CAD build for the part. Positions are in the model's coordinates, mm. A direction names the side the tool comes from. Give positions to 0.01 mm unless a question says otherwise; leave off trailing zeros. Loops run counter-clockwise (first coordinate to the right, second up) from the corner with the lowest first, then second, coordinate; pieces in that order, holes last. Notation, with made-up numbers: M -35.75,58 L -2.75,58 A28 ccw -2.75,92 Z; hole C -20.5,0 d11. An arc over 180 degrees is marked long. One line per question, with ' | ' between items.
```python
from build123d import *

# Parameters (mm, degrees)
EXTRUDE_1_DEPTH     = 300
CUT_EXTRUDE_1_DEPTH = 305.46017802


with BuildPart() as part:
    # 草图1 → 凸台-拉伸1 (new body)
    with BuildSketch(Plane(origin=(0, 0, 0), x_dir=(1, 0, 0), z_dir=(0, 1, 0))):
        Polygon((0, 0), (0, 50), (14, 50), (14, 48), (2, 48), (2, 2), (14, 2), (14, 0), align=None)
    extrude(amount=EXTRUDE_1_DEPTH)

    # 草图2 → 切除-拉伸1 (cut, through all)
    with BuildSketch(Plane.ZY):
        with BuildLine():
            Line((-7, 274), (-7, 26))
            ThreePointArc((-7, 26), (-25, 8), (-43, 26))
            Line((-43, 26), (-43, 274))
            ThreePointArc((-43, 274), (-25, 292), (-7, 274))
        make_face()
    extrude(amount=-CUT_EXTRUDE_1_DEPTH, mode=Mode.SUBTRACT)


solid = part.part
```
Item 1: 3-axis set-ups, long thin cutter, end or side, ignore diameter. For faces 1 (the flat face through (8, 148, -2)), 2 (the cylindrical face through (1, 8, -25)), 3 (the flat face through (7, 148, 0)): which of +Z, -Z, +X, -X, +Y, -Y reach the whole face in a straight line?
Conclusion:
face 1: +X, +Y, -Y | face 2: +X, -X | face 3: +Z, +X, -X, +Y, -Y
Item 2: Mould opens along Y. For faces 4 (the flat face through (8, 148, -48)), 5 (the flat face through (1.8, 300, -23.3)), 6 (the cylindrical face through (1, 292, -25)), 7 (the flat face through (1.8, 0, -23.3)) say: pulls with the +Y half, pulls with the -Y half, needs draft (parallel to the pull), parting line crosses it, or undercut.
Conclusion:
face 4: needs draft | face 5: pulls with the +Y half | face 6: undercut | face 7: pulls with the -Y half
Item 3: Saw through at B-B on y = 253. Give the cut face in (x, z).
Conclusion:
outline: M 0,-50 L 14,-50 L 14,-48 L 2,-48 L 2,-43 L 0,-43 Z; M 0,-7 L 2,-7 L 2,-2 L 14,-2 L 14,0 L 0,0 Z
Item 4: Drill centre lines: line 1 along Z through (x, y) = (8.75, 268); line 2 along Z through (x, y) = (1, 80); line 3 along Y through (x, z) = (1.5, -22). Where is each one in solid material? Low to high. Write a range as [from, to].
Conclusion:
line 1: [-50, -48], [-2, 0] | line 2: [-50, -43], [-7, 0] | line 3: [0, 8.25], [291.75, 300]
Item 5: Saw through at C-C on z = -25. Give the cut face in (x, y).
Conclusion:
outline: M 0,0 L 2,0 L 2,8 L 0,8 Z; M 0,292 L 2,292 L 2,300 L 0,300 Z
Item 6: Saw through at D-D on y = 23.5. Give the cut face in (x, z).
Conclusion:
outline: M 0,-50 L 14,-50 L 14,-48 L 2,-48 L 2,-42.83 L 0,-42.83 Z; M 0,-7.17 L 2,-7.17 L 2,-2 L 14,-2 L 14,0 L 0,0 Z
Item 7: Saw through at A-A on x = 8.5. Give the cut face in (y, z).
Conclusion:
outline: M 0,-50 L 300,-50 L 300,-48 L 0,-48 Z; M 0,-2 L 300,-2 L 300,0 L 0,0 Z
